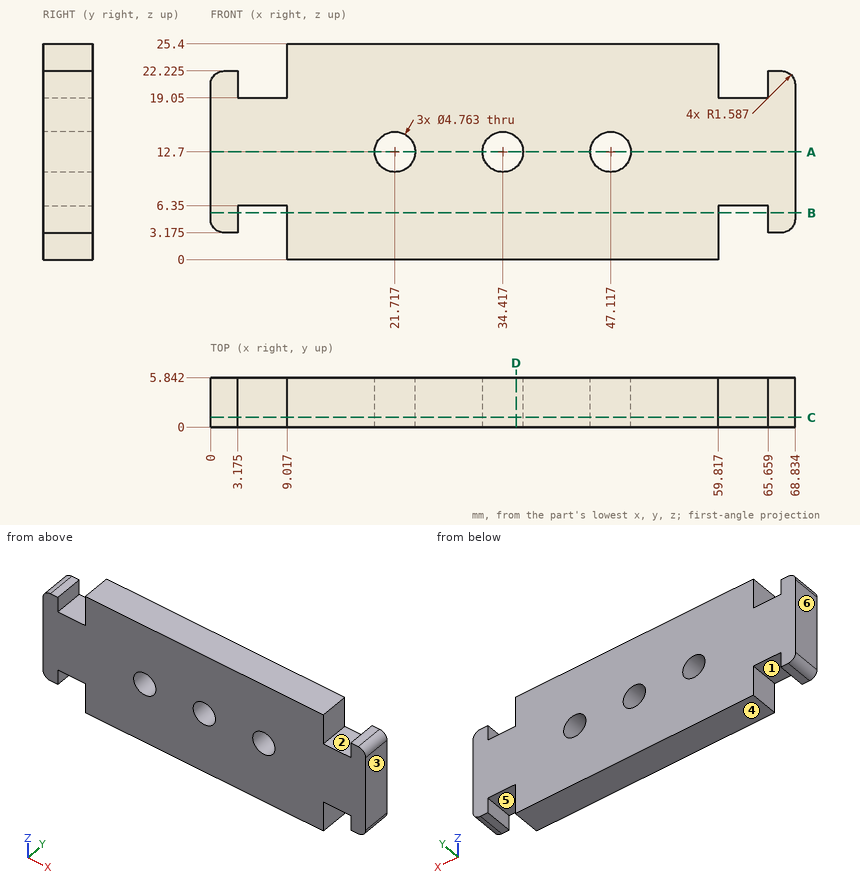
The figure shows three views and two pictorial views of one solid part (mm, origin at its lowest corner). Answer the questions. A direction names the side the tool comes from. Round coordinates to 2 decimals unless told otherwise and drop trailing zeros. Order: outer loops, then holes, each group sorted by start corner. A loop starts at its lowest first (then second) coordinate and runs counter-clockwise, first axis right, second up. Notation, with made-up numbers: (-29, -10.5) - (30, -10.5) arc R22 ccw to (30, 23.5) - close; hole circle Ø10 at (-1.75, 21.25). An arc over 180 degrees is marked (long way). Write item = value, one per line. Start each with the question number.
1) For the marked faces 1, 2 and 3, determine the directions among +Z, -Z, +X, -X, +Y, -Y from which every point of the face is accessible in a straight line to the end or side of a thin tool.
2) Section D-D, the plane x = 36 is taken. Write down the section's boundary in (y, z).
3) Given pin 1 (1.7 mm diameter, centred on x = 66.5, y = 4.5, fed in from -Z) (1 decimal); pin 2 (1.3 mm diameter, centred on x = 2, y = 2.5, fed in from +Z) (1 decimal); pin 3 (1.8 mm diameter, centred on x = 5, y = 2, fed in from +Z), each flat-ended and moving along its own axis, determine where each tip first touches the part or whether it passes through.
4) Straight lines are drawn through the part: L1, parallel to X at y = 4.6, z = 5 (1 decimal); L2, parallel to X at y = 2.2, z = 12.7 (1 decimal); L3, parallel to X at y = 1.25, z = 21.75 (1 decimal). For each, find the intervals that lie inside material, in ascending order.
5) Section C-C, the plane y = 1.15 is taken. Count the separate pieces of the cut face and the enclosed holes in it, plus the area to 3 significant figures.
6) Section A-A, the plane z = 12.7 is taken. Write down the section's boundary in (x, y) (1 decimal).
7) Section B-B, the plane z = 5.5 is taken. Write down the section's boundary in (x, y) (1 decimal), plus the area to 3 significant figures.
8) For a pull along X with two mould halves and no side action, classify the marked faces 4, 5 and 6 as released by +X, released by -X, zero draft, split by the parting line, or undercut.
Results list:
q1.face_1 = -Z, +Y, -Y
q1.face_2 = +Z, +Y, -Y
q1.face_3 = +Z, -Z, +X, +Y, -Y
q2.outline = (0, 0) - (5.84, 0) - (5.84, 10.92) - (0, 10.92) - close; (0, 14.48) - (5.84, 14.48) - (5.84, 25.4) - (0, 25.4) - close
q3.pin_1 = 3.2
q3.pin_2 = 22.2
q3.pin_3 = 19.05
q4.L1 = 0 to 3.2, 9 to 59.8, 65.7 to 68.8
q4.L2 = 0 to 19.3, 24.1 to 32, 36.8 to 44.7, 49.5 to 68.8
q4.L3 = 0.5 to 3.2, 9 to 59.8, 65.7 to 68.4
q5.separate_pieces = 1
q5.enclosed_holes = 3
q5.area = 1,500 mm^2
q6.outline = (0, 0) - (19.3, 0) - (19.3, 5.8) - (0, 5.8) - close; (24.1, 0) - (32, 0) - (32, 5.8) - (24.1, 5.8) - close; (36.8, 0) - (44.7, 0) - (44.7, 5.8) - (36.8, 5.8) - close; (49.5, 0) - (68.8, 0) - (68.8, 5.8) - (49.5, 5.8) - close
q7.outline = (0, 0) - (3.2, 0) - (3.2, 5.8) - (0, 5.8) - close; (9, 0) - (59.8, 0) - (59.8, 5.8) - (9, 5.8) - close; (65.7, 0) - (68.8, 0) - (68.8, 5.8) - (65.7, 5.8) - close
q7.area = 334 mm^2
q8.face_4 = zero draft
q8.face_5 = undercut
q8.face_6 = released by -X
